Input: part model. Units: mm. Frame: model coordinates. Face numbers are marked on the shaded views. A direction names the side the tool comes from. Give positions to 0.01 mm unless a question says otherwise; leave off trailing zeros. Write each loop counter-clockwise with the first axis right and the second up, starting at its lowest first coordinate (ties: lowest second). Pieces come first, ordered by that corner, then holes. Notation, with made-up numbers: (25.25, -25.5) -> (81.25, -25.5) arc R29 ccw to (81.25, 11.5) -> close; hole circle Ø5 at (-12.5, 1). An arc over 180 degrees is marked (long way). Answer as a JSON object with one key per item and string values. Group by question number.
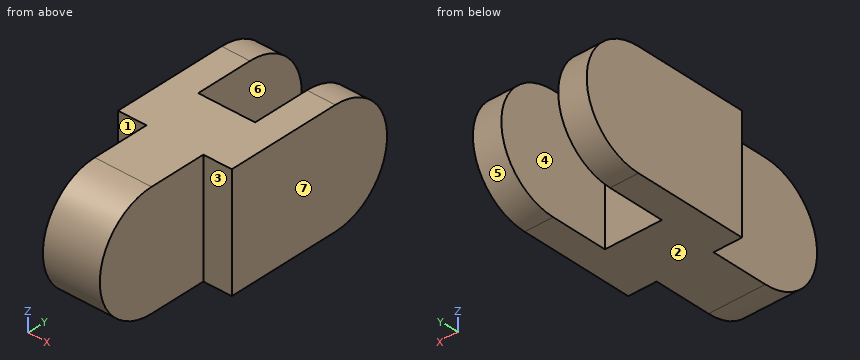
from build123d import *

# Parameters (mm, degrees)
SKETCH_1_W          = 16
SKETCH_1_H          = 16
EXTRUDE_1_DEPTH     = 40
CUT_EXTRUDE_1_DEPTH = 40
CUT_EXTRUDE_START   = -4
CUT_EXTRUDE_2_DEPTH = 4
CUT_EXTRUDE_3_DEPTH = 4
CUT_EXTRUDE_7_DEPTH = 44.8178046
CUT_EXTRUDE_8_DEPTH = 4


with BuildPart() as part:
    # 草图1 → 凸台-拉伸1 (new body)
    with BuildSketch(Plane(origin=(0, 0, 0), x_dir=(1, 0, 0), z_dir=(0, 1, 0))):
        Rectangle(SKETCH_1_W, SKETCH_1_H)
    extrude(amount=EXTRUDE_1_DEPTH)

    # 草图2 → 切除-拉伸1 (cut)
    with BuildSketch(Plane(origin=(8, 0, 0), x_dir=(0, 0, -1), z_dir=(1, 0, 0))):
        with BuildLine():
            Line((-8, 8), (-8, -6.748551072))
            Line((-8, -6.748551072), (8, -6.748551072))
            Line((8, -6.748551072), (8, 8))
            ThreePointArc((8, 8), (0, 0), (-8, 8))
        make_face()
    extrude(amount=-CUT_EXTRUDE_1_DEPTH, mode=Mode.SUBTRACT)

    # 草图4 → 切除-拉伸2 (cut)
    with BuildSketch(Plane.ZY.offset(8).offset(CUT_EXTRUDE_START)):
        with BuildLine():
            Line((-8, 8), (-8, 16))
            Line((-8, 16), (8, 16))
            Line((8, 16), (8, 8))
            ThreePointArc((8, 8), (0, 0), (-8, 8))
        make_face()
    extrude(amount=CUT_EXTRUDE_2_DEPTH, mode=Mode.SUBTRACT)

    # 草图5 → 切除-拉伸3 (cut)
    with BuildSketch(Plane(origin=(8, 0, 0), x_dir=(0, 0, -1), z_dir=(1, 0, 0))):
        with BuildLine():
            Line((-8, 8), (-8, 16))
            Line((-8, 16), (8, 16))
            Line((8, 16), (8, 8))
            ThreePointArc((8, 8), (0, 0), (-8, 8))
        make_face()
    extrude(amount=-CUT_EXTRUDE_3_DEPTH, mode=Mode.SUBTRACT)

    # 草图8 → 切除-拉伸7 (cut, through all)
    with BuildSketch(Plane(origin=(8, 0, 0), x_dir=(0, 0, -1), z_dir=(1, 0, 0))):
        with BuildLine():
            Line((-8, 32), (-8, 44.090265963))
            Line((-8, 44.090265963), (8, 44.090265963))
            Line((8, 44.090265963), (8, 32))
            ThreePointArc((8, 32), (0, 40), (-8, 32))
        make_face()
    extrude(amount=-CUT_EXTRUDE_7_DEPTH, mode=Mode.SUBTRACT)

    # 草图7 → 切除-拉伸8 (cut, symmetric)
    with BuildSketch(Plane(origin=(0, 0, 0), x_dir=(0, 0, -1), z_dir=(1, 0, 0))):
        with BuildLine():
            Line((-8, 32), (-8, 24))
            Line((-8, 24), (8, 24))
            Line((8, 24), (8, 32))
            ThreePointArc((8, 32), (0, 40), (-8, 32))
        make_face()
    extrude(amount=CUT_EXTRUDE_8_DEPTH, both=True, mode=Mode.SUBTRACT)


solid = part.part
1. Mould query, pull axis X, two halves, no side actions, for the marked faces 5, 6 and 7. Classes: pulls with the +X half, pulls with the -X half, needs draft (parallel to the pull), parting line crosses it, or undercut.
2. Reachability of the marked faces 1, 2, 3 and 4 from +Z, -Z, +X, -X, +Y, -Y: full face, straight path, thin tool, end or side. Return the list, or none.
3. Section B-B (y = 35). Return the cut outline in (x, z), plus the area to 3 significant figures.
4. Contact query for flat-ended pins moving along their axis: pin 1 Ø8 at (y, z) = (7, 1.5) entering from -X; pin 2 Ø4.5 at (x, z) = (7, 3) entering from -Y; pin 3 Ø4 at (x, z) = (1.5, 4) entering from +Y. Output: stop coordinate, or through.
5. Section D-D (y = 7). Return the cut outline in (x, z), plus the area to 3 significant figures.
6. Line query: line 1 (X direction, y = 25, z = -6.75); line 2 (X direction, y = 2.5, z = -3); line 3 (Y direction, x = -2.75, z = 0). Output: solid intervals per line, ascending.
7. Section A-A (z = 0). Return the cut outline in (x, y), plus the area to 3 significant figures.
8. Section C-C (x = -3.25). Return the cut outline in (y, z), plus the area to 3 significant figures.
Working result:
{
 "1": {"face 5": "needs draft", "face 6": "undercut", "face 7": "pulls with the +X half"},
 "2": {"face 1": "+Z, -Z, -X, -Y", "face 2": "-Z, +X, -X, +Y, -Y", "face 3": "+Z, -Z, +X, -Y", "face 4": "+Z, -Z, +Y"},
 "3": {"outline": "(-8, -7.42) -> (-4, -7.42) -> (-4, 7.42) -> (-8, 7.42) -> close; (4, -7.42) -> (8, -7.42) -> (8, 7.42) -> (4, 7.42) -> close", "area": "119 mm^2"},
 "4": {"pin 1": "stops at x = -4", "pin 2": "stops at y = 16", "pin 3": "stops at y = 24"},
 "5": {"outline": "(-4, -7.94) -> (4, -7.94) -> (4, 7.94) -> (-4, 7.94) -> close", "area": "127 mm^2"},
 "6": {"line 1": "x = -8 to -4, 4 to 8", "line 2": "x = -4 to 4", "line 3": "y = 0 to 24"},
 "7": {"outline": "(-8, 16) -> (-4, 16) -> (-4, 0) -> (4, 0) -> (4, 16) -> (8, 16) -> (8, 40) -> (4, 40) -> (4, 24) -> (-4, 24) -> (-4, 40) -> (-8, 40) -> close", "area": "384 mm^2"},
 "8": {"outline": "(8, -8) -> (24, -8) -> (24, 8) -> (8, 8) arc R8 ccw to start", "area": "357 mm^2"}
}
